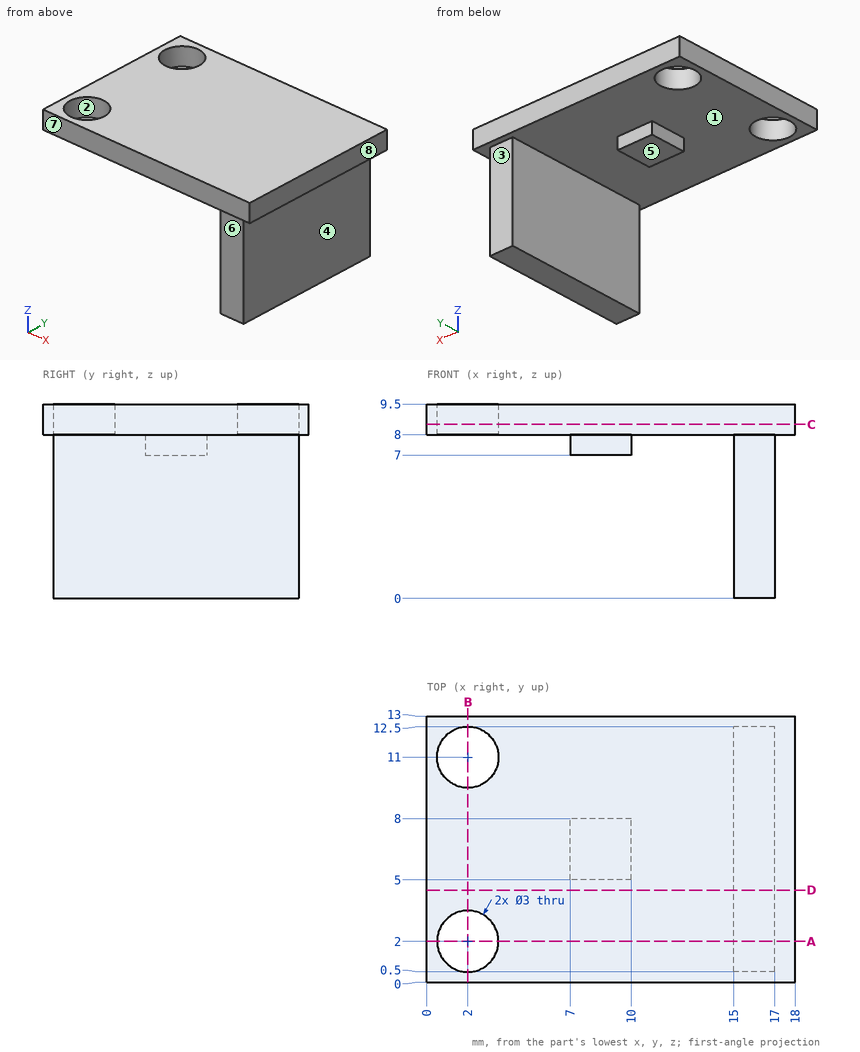
For this review, use the dimensioned drawing (mm, ordinates from the lowest corner) and the shaded views. A direction names the side the tool comes from. Coordinates: 2 decimals unless noted, no trailing zeros. Loops run counter-clockwise (first coordinate to the right, second up) from the corner with the lowest first, then second, coordinate; pieces in that order, holes last. Notation, with made-up numbers: (85, 63.25) - (131, 63.25) arc R8 ccw to (131, 72.25) - close; hole circle Ø6 at (66, -38.75). An arc over 180 degrees is marked (long way). Use CSV: the item, a comma, the result in double quotes. Start each with the question number.
1) Consider section C-C on z = 8.5. Write out the cut boundary in (x, y), then the cut area to 3 significant figures.
2) Consider section B-B on x = 2. Write out the cut boundary in (y, z), then the cut area to 3 significant figures.
3) Wall thickness on L1, parallel to Y at x = 2, z = 8.8; L2, parallel to X at y = 2, z = 8.65; L3, parallel to Z at x = 3, y = 9.75: over which ranges is each line inside the solid? List them lowest first. Write a range as from..to.
4) For pin 1 Ø4 at (x, y) = (11, 9) entering from -Z; pin 2 Ø2 at (x, z) = (16, 2) entering from -Y; pin 3 Ø0.8 at (y, z) = (6.5, 7.5) entering from -X; pin 4 Ø2.5 at (x, y) = (2, 2) entering from +Z, all flat-tipped, find the tip position at first contact; note any pin that passes through.
5) Consider section D-D on y = 4.5. Write out the cut boundary in (x, z).
6) The part is to be moulded in two halves that separate along Y. For the marked faces 1, 2 and 3, say which applies: +Y half, -Y half, draft (parallel to the pull), parting line (faces both ways), or undercut.
7) Consider section A-A on y = 2. Write out the cut boundary in (x, z).
8) Tool access review of the marked faces 4, 5, 6, 7 and 8: name each direction out of +Z, -Z, +X, -X, +Y, -Y from which nothing blocks a thin tool from reaching the whole face with its end or side.
Geometry says:
1,outline,"(0, 0) - (18, 0) - (18, 13) - (0, 13) - close; hole circle Ø3 at (2, 2); hole circle Ø3 at (2, 11)"
1,area,"220 mm^2"
2,outline,"(0, 8) - (0.5, 8) - (0.5, 9.5) - (0, 9.5) - close; (3.5, 8) - (9.5, 8) - (9.5, 9.5) - (3.5, 9.5) - close; (12.5, 8) - (13, 8) - (13, 9.5) - (12.5, 9.5) - close"
2,area,"10.5 mm^2"
3,L1,"0..0.5, 3.5..9.5, 12.5..13"
3,L2,"0..0.5, 3.5..18"
3,L3,"8..9.5"
4,pin 1,"z = 7"
4,pin 2,"y = 0.5"
4,pin 3,"x = 7"
4,pin 4,"through"
5,outline,"(0, 8) - (15, 8) - (15, 0) - (17, 0) - (17, 8) - (18, 8) - (18, 9.5) - (0, 9.5) - close"
6,face 1,"draft"
6,face 2,"undercut"
6,face 3,"+Y half"
7,outline,"(0, 8) - (0.5, 8) - (0.5, 9.5) - (0, 9.5) - close; (3.5, 8) - (15, 8) - (15, 0) - (17, 0) - (17, 8) - (18, 8) - (18, 9.5) - (3.5, 9.5) - close"
8,face 4,"-Z, +X, +Y, -Y"
8,face 5,"-Z, -X, +Y, -Y"
8,face 6,"-Z, +X, -X, -Y"
8,face 7,"+Z, -Z, +X, -X, -Y"
8,face 8,"+Z, -Z, +X, +Y, -Y"
